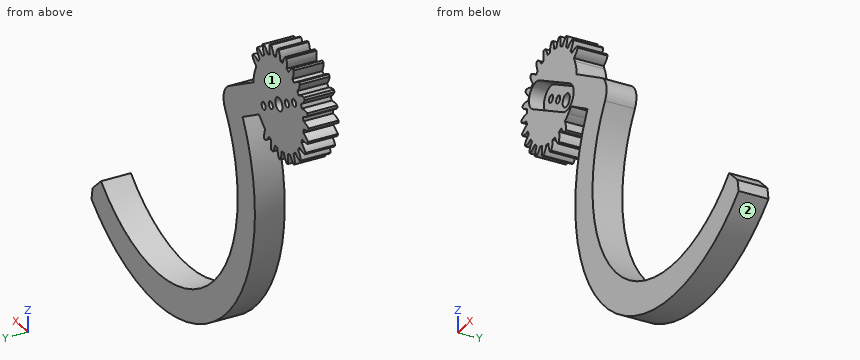
from build123d import *

# Parameters (mm, degrees)
CROQUIS3_R              = 1.75
SALIENTE_EXTRUIR2_DEPTH = 8
CROQUIS4_R              = 1
CORTAR_EXTRUIR1_DEPTH   = 8
CORTAR_EXTRUIR2_DEPTH   = 4


with BuildPart() as part:
    # Croquis3 → Saliente-Extruir2 (new body)
    with BuildSketch(Plane(origin=(0, 0, 0), x_dir=(1, 0, 0), z_dir=(0, 1, 0))):
        with BuildLine():
            Line((87.111019212, 63.804032696), (91.223264764, 67.638763711))
            Line((91.223264764, 67.638763711), (91.815621149, 70.950831381))
            ThreePointArc((91.815621149, 70.950831381), (29.87732987, 72.940785596), (17.735388738, 12.171672472))
            Line((17.735388738, 12.171672472), (9.721894551, 7.515983209))
            ThreePointArc((9.721894551, 7.515983209), (9.056743368, 8.17044576), (8.33477019, 8.76163275))
            ThreePointArc((8.33477019, 8.76163275), (7.527702463, 9.464052948), (6.66170644, 10.092386728))
            ThreePointArc((6.66170644, 10.092386728), (7.120443737, 11.359558341), (7.251125308, 12.700858505))
            ThreePointArc((7.251125308, 12.700858505), (6.978446869, 12.852700273), (6.702590326, 12.9986887))
            ThreePointArc((6.702590326, 12.9986887), (5.648855639, 12.158565486), (4.835962342, 11.083684892))
            ThreePointArc((4.835962342, 11.083684892), (4.333654022, 11.289554703), (3.822612402, 11.472673489))
            ThreePointArc((3.822612402, 11.472673489), (3.937750458, 12.815397225), (3.716825134, 14.144816574))
            ThreePointArc((3.716825134, 14.144816574), (3.414138446, 14.220910086), (3.109896902, 14.290527151))
            ThreePointArc((3.109896902, 14.290527151), (2.349191787, 13.184063868), (1.802512181, 11.957656643))
            ThreePointArc((1.802512181, 11.957656643), (1.264036574, 12.02650465), (0.723013645, 12.071116511))
            ThreePointArc((0.723013645, 12.071116511), (0.486705992, 13.397887968), (-0.07077053, 14.624828769))
            ThreePointArc((-0.07077053, 14.624828769), (-0.382837869, 14.619988378), (-0.694730857, 14.608489793))
            ThreePointArc((-0.694730857, 14.608489793), (-1.187230257, 13.354054404), (-1.353776206, 12.016733855))
            ThreePointArc((-1.353776206, 12.016733855), (-1.891722877, 11.943868181), (-2.425857296, 11.846932892))
            ThreePointArc((-2.425857296, 11.846932892), (-2.997506682, 13.067334786), (-3.8535433, 14.108183052))
            ThreePointArc((-3.8535433, 14.108183052), (-4.153724416, 14.022738622), (-4.452013856, 13.930907997))
            ThreePointArc((-4.452013856, 13.930907997), (-4.603059976, 12.591748233), (-4.417806982, 11.256890513))
            ThreePointArc((-4.417806982, 11.256890513), (-4.918564541, 11.047276833), (-5.409410071, 10.815400374))
            ThreePointArc((-5.409410071, 10.815400374), (-6.27744423, 11.846264333), (-7.373703462, 12.630087975))
            ThreePointArc((-7.373703462, 12.630087975), (-7.641541509, 12.469862404), (-7.905899467, 12.303957843))
            ThreePointArc((-7.905899467, 12.303957843), (-7.705198765, 10.971335229), (-7.180771513, 9.729908686))
            ThreePointArc((-7.180771513, 9.729908686), (-7.610214159, 9.397831825), (-8.02432049, 9.046816193))
            ThreePointArc((-8.02432049, 9.046816193), (-9.129584328, 9.817890543), (-10.391357918, 10.291273275))
            ThreePointArc((-10.391357918, 10.291273275), (-10.608600176, 10.06718567), (-10.821011096, 9.838513296))
            ThreePointArc((-10.821011096, 9.838513296), (-10.282240991, 8.60324386), (-9.454378332, 7.539849661))
            ThreePointArc((-9.454378332, 7.539849661), (-9.783240259, 7.10794011), (-10.092386728, 6.66170644))
            ThreePointArc((-10.092386728, 6.66170644), (-11.359558341, 7.120443737), (-12.700858505, 7.251125308))
            ThreePointArc((-12.700858505, 7.251125308), (-12.852700273, 6.978446869), (-12.9986887, 6.702590326))
            ThreePointArc((-12.9986887, 6.702590326), (-12.158565486, 5.648855639), (-11.083684892, 4.835962342))
            ThreePointArc((-11.083684892, 4.835962342), (-11.289554703, 4.333654022), (-11.472673489, 3.822612402))
            ThreePointArc((-11.472673489, 3.822612402), (-12.815397225, 3.937750458), (-14.144816574, 3.716825134))
            ThreePointArc((-14.144816574, 3.716825134), (-14.220910086, 3.414138446), (-14.290527151, 3.109896902))
            ThreePointArc((-14.290527151, 3.109896902), (-13.206303836, 2.309507242), (-11.957656643, 1.802512181))
            ThreePointArc((-11.957656643, 1.802512181), (-12.02650465, 1.264036574), (-12.071116511, 0.723013645))
            ThreePointArc((-12.071116511, 0.723013645), (-13.397887968, 0.486705992), (-14.624828769, -0.07077053))
            ThreePointArc((-14.624828769, -0.07077053), (-14.619988378, -0.382837869), (-14.608489793, -0.694730857))
            ThreePointArc((-14.608489793, -0.694730857), (-13.354054404, -1.187230257), (-12.016733855, -1.353776206))
            ThreePointArc((-12.016733855, -1.353776206), (-11.943868181, -1.891722877), (-11.846932892, -2.425857296))
            ThreePointArc((-11.846932892, -2.425857296), (-13.067334786, -2.997506682), (-14.108183052, -3.8535433))
            ThreePointArc((-14.108183052, -3.8535433), (-14.022738622, -4.153724416), (-13.930907997, -4.452013856))
            ThreePointArc((-13.930907997, -4.452013856), (-12.591748233, -4.603059976), (-11.256890513, -4.417806982))
            ThreePointArc((-11.256890513, -4.417806982), (-11.047276833, -4.918564541), (-10.815400374, -5.409410071))
            ThreePointArc((-10.815400374, -5.409410071), (-11.846264333, -6.27744423), (-12.630087975, -7.373703462))
            ThreePointArc((-12.630087975, -7.373703462), (-12.469862404, -7.641541509), (-12.303957843, -7.905899467))
            ThreePointArc((-12.303957843, -7.905899467), (-10.971335229, -7.705198765), (-9.729908686, -7.180771513))
            ThreePointArc((-9.729908686, -7.180771513), (-9.397831825, -7.610214159), (-9.046816193, -8.02432049))
            ThreePointArc((-9.046816193, -8.02432049), (-9.817890543, -9.129584328), (-10.291273275, -10.391357918))
            ThreePointArc((-10.291273275, -10.391357918), (-10.06718567, -10.608600176), (-9.838513296, -10.821011096))
            ThreePointArc((-9.838513296, -10.821011096), (-8.60324386, -10.282240991), (-7.539849661, -9.454378332))
            ThreePointArc((-7.539849661, -9.454378332), (-7.10794011, -9.783240259), (-6.66170644, -10.092386728))
            ThreePointArc((-6.66170644, -10.092386728), (-7.120443737, -11.359558341), (-7.251125308, -12.700858505))
            ThreePointArc((-7.251125308, -12.700858505), (-6.978446869, -12.852700273), (-6.702590326, -12.9986887))
            ThreePointArc((-6.702590326, -12.9986887), (-5.648855639, -12.158565486), (-4.835962342, -11.083684892))
            ThreePointArc((-4.835962342, -11.083684892), (-4.333654022, -11.289554703), (-3.822612402, -11.472673489))
            ThreePointArc((-3.822612402, -11.472673489), (-3.937750458, -12.815397225), (-3.716825134, -14.144816574))
            ThreePointArc((-3.716825134, -14.144816574), (-3.414138446, -14.220910086), (-3.109896902, -14.290527151))
            ThreePointArc((-3.109896902, -14.290527151), (-2.309507242, -13.206303836), (-1.802512181, -11.957656643))
            ThreePointArc((-1.802512181, -11.957656643), (-1.264036574, -12.02650465), (-0.723013645, -12.071116511))
            ThreePointArc((-0.723013645, -12.071116511), (-0.486705992, -13.397887968), (0.07077053, -14.624828769))
            ThreePointArc((0.07077053, -14.624828769), (0.382837869, -14.619988378), (0.694730857, -14.608489793))
            ThreePointArc((0.694730857, -14.608489793), (1.187230257, -13.354054404), (1.353776206, -12.016733855))
            ThreePointArc((1.353776206, -12.016733855), (1.891722877, -11.943868181), (2.425857296, -11.846932892))
            ThreePointArc((2.425857296, -11.846932892), (2.997506682, -13.067334786), (3.8535433, -14.108183052))
            ThreePointArc((3.8535433, -14.108183052), (4.153724416, -14.022738622), (4.452013856, -13.930907997))
            ThreePointArc((4.452013856, -13.930907997), (4.603059976, -12.591748233), (4.417806982, -11.256890513))
            ThreePointArc((4.417806982, -11.256890513), (4.918564541, -11.047276833), (5.409410071, -10.815400374))
            ThreePointArc((5.409410071, -10.815400374), (6.27744423, -11.846264333), (7.373703462, -12.630087975))
            ThreePointArc((7.373703462, -12.630087975), (7.641541509, -12.469862404), (7.905899467, -12.303957843))
            ThreePointArc((7.905899467, -12.303957843), (7.705198765, -10.971335229), (7.180771513, -9.729908686))
            ThreePointArc((7.180771513, -9.729908686), (7.610214159, -9.397831825), (8.02432049, -9.046816193))
            ThreePointArc((8.02432049, -9.046816193), (9.129584328, -9.817890543), (10.391357918, -10.291273275))
            Line((10.391357918, -10.291273275), (10.821011096, -9.838513296))
            ThreePointArc((10.821011096, -9.838513296), (10.282240991, -8.60324386), (9.454378332, -7.539849661))
            ThreePointArc((9.454378332, -7.539849661), (9.783240259, -7.10794011), (10.092386728, -6.66170644))
            ThreePointArc((10.092386728, -6.66170644), (11.359558341, -7.120443737), (12.700858505, -7.251125308))
            ThreePointArc((12.700858505, -7.251125308), (12.852700273, -6.978446869), (12.9986887, -6.702590326))
            ThreePointArc((12.9986887, -6.702590326), (12.158565486, -5.648855639), (11.083684892, -4.835962342))
            ThreePointArc((11.083684892, -4.835962342), (11.289554703, -4.333654022), (11.472673489, -3.822612402))
            ThreePointArc((11.472673489, -3.822612402), (12.166604466, -1.858471402), (12.448632794, 0.205469027))
            Line((12.448632794, 0.205469027), (24.597080908, 7.219378816))
            ThreePointArc((24.597080908, 7.219378816), (26.952693775, 10.356600271), (26.318983455, 14.228225469))
            ThreePointArc((26.318983455, 14.228225469), (34.708358258, 66.001642936), (87.111019212, 63.804032696))
        make_face()
        with Locations(Location((0, 0, 0), (0, 0, 270))):
            Circle(CROQUIS3_R, mode=Mode.SUBTRACT)
    extrude(amount=SALIENTE_EXTRUIR2_DEPTH)

    # Croquis4 → Cortar-Extruir1 (cut)
    with BuildSketch(Plane(origin=(0, 8, 0), x_dir=(1, 0, 0), z_dir=(0, 1, 0))):
        with Locations(Location((3.943679518, 2.167346732, 0), (0, 0, 270))):
            Circle(CROQUIS4_R)
        with Locations(Location((-3.943679518, -2.167346732, 0), (0, 0, 270))):
            Circle(CROQUIS4_R)
        with Locations(Location((7.449172424, 4.09387716, 0), (0, 0, 270))):
            Circle(CROQUIS4_R)
        with Locations(Location((-7.449172424, -4.09387716, 0), (0, 0, 270))):
            Circle(CROQUIS4_R)
    extrude(amount=-CORTAR_EXTRUIR1_DEPTH, mode=Mode.SUBTRACT)

    # Croquis5 → Cortar-Extruir2 (cut)
    with BuildSketch(Plane.XZ):
        with BuildLine():
            Line((-5.763458299, 7.161183452), (9.134886548, -1.026570868))
            ThreePointArc((9.134886548, -1.026570868), (10.516478716, -5.779591285), (5.763458299, -7.161183452))
            Line((5.763458299, -7.161183452), (-9.134886548, 1.026570868))
            ThreePointArc((-9.134886548, 1.026570868), (-10.516478716, 5.779591285), (-5.763458299, 7.161183452))
        make_face()
    extrude(amount=-CORTAR_EXTRUIR2_DEPTH, mode=Mode.SUBTRACT)


solid = part.part
Design review of the part built by this model. Coordinates are the model's own, in mm. Face numbers are marked on the shaded views. Give positions to 0.01 mm unless a question says otherwise; leave off trailing zeros. Order: outer loops, then holes, each group sorted by start corner. A loop starts at its lowest first (then second) coordinate and runs counter-clockwise, first axis right, second up.
1. For pin 1 Ø1.6 at (x, z) = (7.45, -4.09) entering from -Y; pin 2 Ø3 at (x, z) = (-3.94, 2.17) entering from -Y; pin 3 Ø3 at (y, z) = (4.5, 2) entering from -X; pin 4 Ø1 at (x, y) = (77.5, 7) entering from +Z, all flat-tipped, find the tip position at first contact; note any pin that passes through.
Solution:
pin 1: passes through
pin 2: stops at y = 4
pin 3: stops at x = -14.62
pin 4: stops at z = -70.38
2. Add section A-A, the plane x = 22. State the section outline as (y, z) points.
Solution:
outline: (0, -65.03) - (8, -65.03) - (8, -47.27) - (0, -47.27) - close; (0, -23.51) - (8, -23.51) - (8, -5.72) - (0, -5.72) - close
3. Add section B-B, the plane x = 47.5. State the section outline as (y, z) points.
Solution:
outline: (0, -81.75) - (8, -81.75) - (8, -72.97) - (0, -72.97) - close
4. Mouldability with a two-part tool opening along Z and no side actions: class the marked faces 1 and 2 as +Z half, -Z half, draft (parallel to the pull), parting line (faces both ways), or undercut.
Solution:
face 1: draft
face 2: undercut
5. To check wall thickness, follow L1, parallel to Z at x = -1.5, y = 1; L2, parallel to X at y = 6, z = -11; L3, parallel to X at y = 7.25, z = -9. State the ranges of each line that lie inside material, in increasing order.
Solution:
L1: z = -12 to -3.17, 4.82 to 12
L2: x = -7.71 to -5.53, -5.02 to 7.03, 15.72 to 27.07
L3: x = -10.5 to 8.08, 12.28 to 26.4
6. Add section C-C, the plane z = -34. State the section outline as (x, y) points, then the cut area to 3 significant figures.
Solution:
outline: (11.76, 0) - (20.2, 0) - (20.2, 8) - (11.76, 8) - close
area: 67.5 mm2
